Answer from the drawing. Dimensions are ordinates in mm from the lowest x, y and z of the part. A direction names the side the tool comes from. Round coordinates to 2 decimals unless told otherwise and drop trailing zeros. Write each loop counter-clockwise with the first axis right and the second up, starting at its lowest first coordinate (ties: lowest second). Pieces come first, ordered by that corner, then holes. Notation, with made-up numbers: (-26, -10.75) - (-11, -10.75) arc R21 ccw to (-11, 15.25) - close; hole circle Ø5 at (12, -2). An arc over 180 degrees is marked (long way). Answer as a JSON object with one key per item and string values.
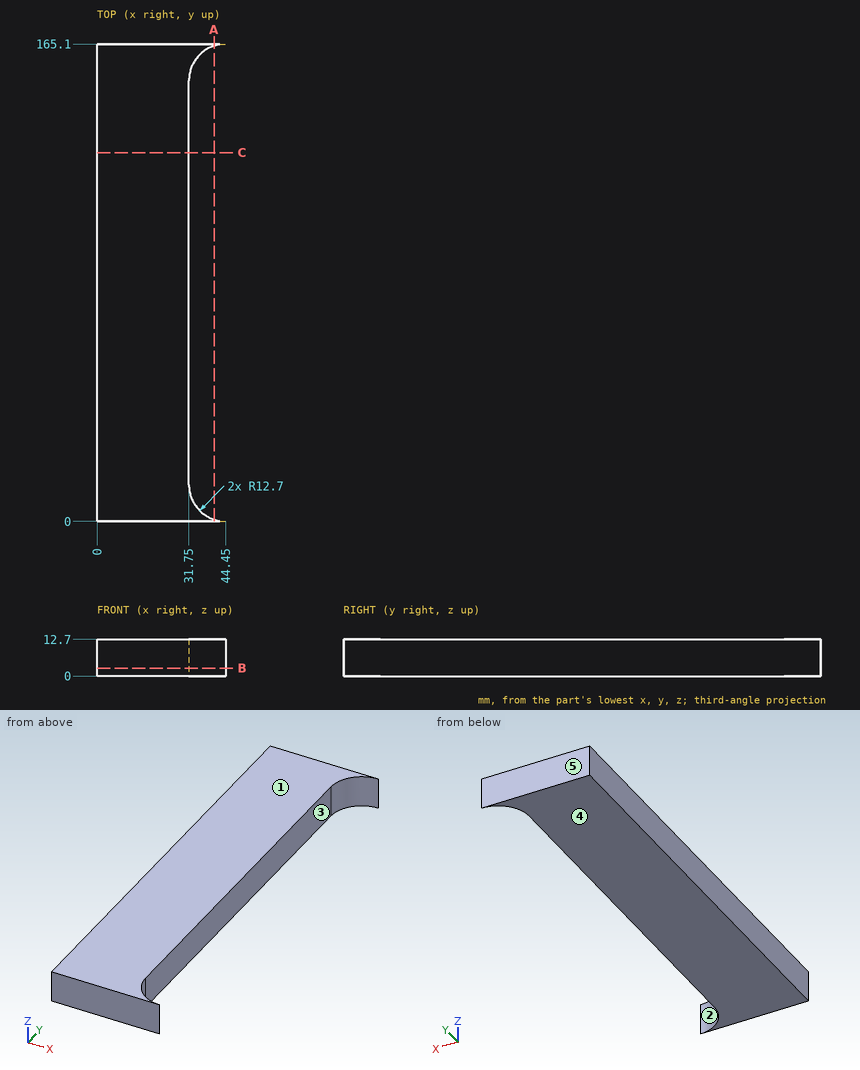
Item 1: A cutting plane is placed at C-C (y = 127.5). Write down the section's boundary in (x, z).
Results found:
{"outline": "(0, 0) - (31.75, 0) - (31.75, 12.7) - (0, 12.7) - close"}
Item 2: A cutting plane is placed at B-B (z = 2.75). Write down the section's boundary in (x, y), and give its area (3 significant figures).
Results found:
{"outline": "(0, 0) - (44.45, 0) arc R12.7 cw to (31.75, 12.7) - (31.75, 152.4) arc R12.7 cw to (44.45, 165.1) - (0, 165.1) - close", "area": "5,310 mm²"}
Item 3: This flat-tipped pin is pushed along its axis until it touches: P1, Ø2, axis at x = 30.5, y = 90, coming from the -Z side. Where does it stop, or does it pass through?
Results found:
{"P1": "z = 0"}
Item 4: Consider line 1 along X through (y, z) = (27.5, 2); line 2 along Y through (x, z) = (34, 12.25); line 3 along Y through (x, z) = (37, 5.75). Determine where each line is inside the solid, lowest interval first.
Results found:
{"line 1": "0 to 31.75", "line 2": "0 to 5.48, 159.62 to 165.1", "line 3": "0 to 2.41, 162.69 to 165.1"}
Item 5: For the marked faces 1 and 2, determine the directions among +Z, -Z, +X, -X, +Y, -Y from which every point of the face is accessible in a straight line to the end or side of a thin tool.
Results found:
{"face 1": "+Z, +X, -X, +Y, -Y", "face 2": "+Z, -Z, +X"}
Item 6: Determine the mould class of the marked faces 3, 4 and 5 for opening direction Y: pulls with the +Y half, pulls with the -Y half, needs draft (parallel to the pull), parting line crosses it, or undercut.
Results found:
{"face 3": "undercut", "face 4": "needs draft", "face 5": "pulls with the +Y half"}
Item 7: A cutting plane is placed at A-A (x = 40.5). Write down the section's boundary in (y, z).
Results found:
{"outline": "(0, 0) - (0.63, 0) - (0.63, 12.7) - (0, 12.7) - close; (164.47, 0) - (165.1, 0) - (165.1, 12.7) - (164.47, 12.7) - close"}
